Work out the finished part from the listing and answer in its coordinate system (mm). Face numbers are marked on the shaded views. A direction names the side the tool comes from. Round coordinates to 2 decimals unless told otherwise and drop trailing zeros. Order: outer loops, then holes, each group sorted by start corner. A loop starts at its lowest first (then second) coordinate and runs counter-clockwise, first axis right, second up. Notation, with made-up numbers: (86, 45) -> (135, 45) arc R20 cw to (135, 67) -> close; hole circle Ø2 at (44.25, -3). An arc over 180 degrees is marked (long way). Use one line per item in the form item = value.
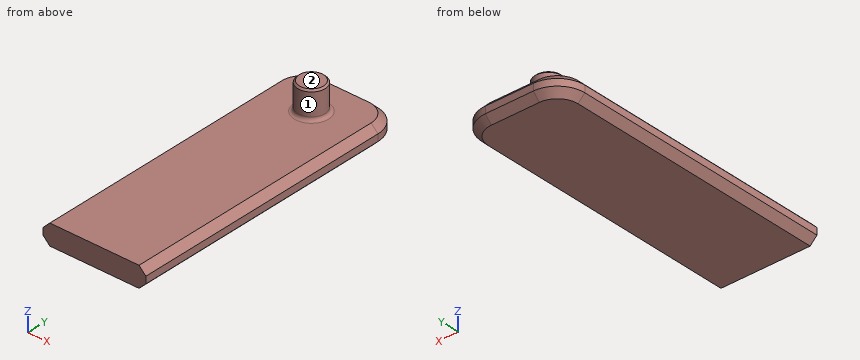
Autodesk Inventor part; units mm, degrees
ref_plane "YZ Plane" through (0, 0, 0) normal (1, 0, 0) x (0, 1, 0)
ref_plane "XZ Plane" through (0, 0, 0) normal (0, 1, 0) x (-1, 0, 0)
ref_plane "XY Plane" through (0, 0, 0) normal (0, 0, 1) x (1, 0, 0)
sketch "Sketch1" plane through (0, 0, 0) normal (0, 0, 1) x (1, 0, 0)
  line L0 (-15, 0) -> (15, 0)
  line L1 (15, 0) -> (15, 85)
  line L2 (15, 85) -> (-15, 85)
  line L3 (-15, 85) -> (-15, 0)
  point P0 (0, 0)
  dimension "d0" = 30
  dimension "d1" = 85
  dimension "d2" = 15
  dimension "d3" = 85
extrude "Extrusion1" add sketch "Sketch1" along normal blind 6
fillet "Fillet1" radius 8 2 edges at (15, 85, 3) (-15, 85, 3)
sketch "Sketch2" plane through (0, 0, 6) normal (0, 0, 1) x (1, 0, 0)
  circle A0 centre (0, 72) radius 4
  line L0 (-15, 0) -> (15, 0)
  point P0 (0, 0)
  dimension "d7" = 72
  dimension "d8" = 8
  dimension "d12" = 0
extrude "Extrusion2" add sketch "Sketch2" along normal blind 8
fillet "Fillet2" radius 1 1 edges at (-4, 72, 6)
chamfer "Chamfer1" distance 0.5 angle 45 1 edges at (-4, 72, 14)
chamfer "Chamfer2" distance 2 angle 45 10 edges at (0, 85, 6) (-12.6569, 82.6569, 6) (-15, 38.5, 6) (12.6569, 82.6569, 6) (15, 38.5, 6) (0, 85, 0) (-12.6569, 82.6569, 0) (-15, 38.5, 0) (12.6569, 82.6569, 0) (15, 38.5, 0)
equation "\"d8\" = d"
equation "\"d\" = 8"
properties part number "reelTab" material "Steel, Mild"
Item 1: Flat-ended cylindrical pins translate along their axes: P1, Ø8, axis at x = -12, y = 32.5, coming from the +Z side; P2, Ø8, axis at y = 53.5, z = 12.5, coming from the +X side. Find the tip coordinate at first contact, or state that the pin passes through.
Findings:
P1 = 6
P2 = through
Item 2: The part is cut by section D-D, the plane y = 44. Give the vertices of the cut face in (x, z).
Findings:
outline = (-15, 2) -> (-13, 0) -> (13, 0) -> (15, 2) -> (15, 4) -> (13, 6) -> (-13, 6) -> (-15, 4) -> close
Item 3: Consider line 1 along Z through (x, y) = (8.75, 14); line 2 along Z through (x, y) = (13.5, 70.5); line 3 along X through (y, z) = (44, 1). Determine where each line is inside the solid, lowest interval first.
Findings:
line_1 = 0 to 6
line_2 = 0.5 to 5.5
line_3 = -14 to 14
Item 4: For the marked faces 1 and 2, determine the directions among +Z, -Z, +X, -X, +Y, -Y from which every point of the face is accessible in a straight line to the end or side of a thin tool.
Findings:
face_1 = +Z
face_2 = +Z, +X, -X, +Y, -Y
Item 5: The part is cut by section C-C, the plane z = 5.25. Give the vertices of the cut face in (x, y).
Findings:
outline = (-13.75, 0) -> (13.75, 0) -> (13.75, 77) arc R6.75 ccw to (7, 83.75) -> (-7, 83.75) arc R6.75 ccw to (-13.75, 77) -> close
Item 6: The part is cut by section A-A, the plane y = 72. Give the vertices of the cut face in (x, z).
Findings:
outline = (-15, 2) -> (-13, 0) -> (13, 0) -> (15, 2) -> (15, 4) -> (13, 6) -> (5, 6) arc R1 cw to (4, 7) -> (4, 13.5) -> (3.5, 14) -> (-3.5, 14) -> (-4, 13.5) -> (-4, 7) arc R1 cw to (-5, 6) -> (-13, 6) -> (-15, 4) -> close
Item 7: The part is cut by section B-B, the plane x = 0. Give the vertices of the cut face in (y, z).
Findings:
outline = (0, 0) -> (83, 0) -> (85, 2) -> (85, 4) -> (83, 6) -> (77, 6) arc R1 cw to (76, 7) -> (76, 13.5) -> (75.5, 14) -> (68.5, 14) -> (68, 13.5) -> (68, 7) arc R1 cw to (67, 6) -> (0, 6) -> close
